Design review of the part built by this model. Coordinates are the model's own, in mm. Face numbers are marked on the shaded views. A direction names the side the tool comes from. Coordinates: 2 decimals unless noted, no trailing zeros. Loops run counter-clockwise (first coordinate to the right, second up) from the corner with the lowest first, then second, coordinate; pieces in that order, holes last. Notation, with made-up numbers: M 89.25,25 L 135.25,25 A21 ccw 135.25,30 Z; hole C 53.5,52.25 d6. An arc over 180 degrees is marked long. Put each result on its own line as item: value. Start each with the question number.
(1) Take a section at A-A, the plane x = 34.1. Give the boundary of the cut face in (y, z).
(2) Take a section at B-B, the plane y = 24.1. Give the boundary of the cut face in (x, z).
(3) Take a section at C-C, the plane x = 40.25. Give the boundary of the cut face in (y, z), then the cut area to 3 significant figures.
(4) For probe 1 along X at (y, z) = (24.1, 1); probe 2 along Y at (x, z) = (38.25, 19); probe 3 along X at (y, z) = (17, 4.25), list the stretches that pass through material, from the lowest coordinate up. Write a range as [from, to].
(5) The part is to be moulded in two halves that separate along X. For the marked faces 1, 2 and 3, say which applies: +X half, -X half, draft (parallel to the pull), parting line (faces both ways), or undercut.
(6) Take a section at D-D, the plane z = 12.5. Give the boundary of the cut face in (x, y), then the cut area to 3 significant figures.
(7) Clearance check with flat-ended pins moving along their axes: pin 1 (1.5 mm diameter, centred on x = 26.5, y = 29.5, fed in from +Z); pin 2 (3 mm diameter, centred on x = 34.1, y = 24.1, fed in from +Z); pin 3 (6 mm diameter, centred on x = 26, y = 26, fed in from +Z); pin 4 (12 mm diameter, centred on x = 26.5, z = 12, fed in from +Y). State where each tip first meets the part, or that it passes through.
(8) For the marked faces 4 and 5, list the 3-axis set-ups (+Z, -Z, +X, -X, +Y, -Y) from which the entire face can be reached by the end or side of a thin tool; tool diameter is ignored.
```python
from build123d import *

# Parameters (mm, degrees)
PAD001_DEPTH            = 20
POCKET001_DEPTH         = 16
HOLE002_D               = 4
HOLE002_CSINK_D         = 7
HOLE002_CSINK_ANGLE     = 90
HOLE003_D               = 4.2
HOLE003_DEPTH           = 25
HOLE003_CSINK_D         = 8.1
HOLE003_CSINK_ANGLE     = 90
BODY001_PLACEMENT_ANGLE = 90


with BuildPart() as part:
    # Sketch004 → Pad001 (new body)
    with BuildSketch(Plane.XZ):
        with BuildLine():
            Line((1, 0), (19, 0))
            ThreePointArc((19, 0), (19.707107, 0.292893), (20, 1))
            Line((20, 1), (20, 2))
            ThreePointArc((20, 2), (19.92388, 2.382683), (19.707107, 2.707107))
            Line((19.707107, 2.707107), (2.707107, 19.707107))
            ThreePointArc((2.707107, 19.707107), (2.382683, 19.92388), (2, 20))
            Line((2, 20), (1, 20))
            Line((1, 20), (1, 0))
        make_face()
    extrude(amount=PAD001_DEPTH)

    # Sketch005 (on Face10 of Pad001) → Pocket001 (cut)
    with BuildSketch(Plane.XZ.offset(18)):
        with BuildLine():
            Line((3, 19), (3, 4))
            ThreePointArc((3, 4), (3.292893, 3.292893), (4, 3))
            Line((4, 3), (19, 3))
            ThreePointArc((20, 2), (19.707107, 2.707107), (19, 3))
            Line((20, 20), (20, 2))
            Line((2, 20), (20, 20))
            ThreePointArc((3, 19), (2.707107, 19.707107), (2, 20))
        make_face()
    extrude(amount=-POCKET001_DEPTH, mode=Mode.SUBTRACT)

    # Hole002 (through all)
    with Locations(Plane(origin=(0, 0, 3), x_dir=(-1, 0, 0), z_dir=(0, 0, 1))):
        with Locations((-11.5, 10)):
            CounterSinkHole(HOLE002_D / 2, HOLE002_CSINK_D / 2, counter_sink_angle=HOLE002_CSINK_ANGLE)

    # Hole003
    with Locations(Plane(origin=(3, 0, 0), x_dir=(0, 0, 1), z_dir=(1, 0, 0))):
        with Locations((12.5, 10)):
            CounterSinkHole(HOLE003_D / 2, HOLE003_CSINK_D / 2, depth=HOLE003_DEPTH, counter_sink_angle=HOLE003_CSINK_ANGLE)


with BuildPart() as part_1:
    # Body001 placement: moved
    add(part.part.moved(Location((24.1, 12.6, 0))).rotate(Axis((24.1, 12.6, 0), (0, 0, 1)), BODY001_PLACEMENT_ANGLE))


solid = part_1.part
```
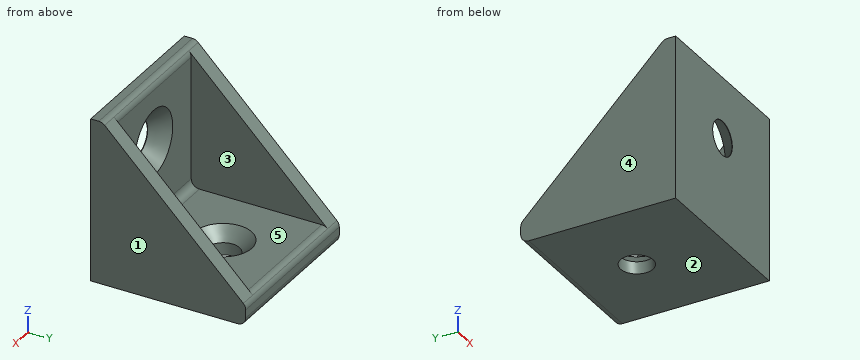
Computed values:
1. outline: M 13.6,0 L 22.1,0 L 22.1,1.5 L 20.6,3 L 16.6,3 A1 cw 15.6,4 L 15.6,8.45 L 13.65,10.4 L 13.6,10.4 Z; M 13.6,14.6 L 13.65,14.6 L 15.6,16.55 L 15.6,19 A1 ccw 14.6,20 L 13.6,20 Z; M 26.1,0 L 31.6,0 A1 ccw 32.6,1 L 32.6,2 A1 ccw 31.6,3 L 27.6,3 L 26.1,1.5 Z
2. outline: M 24.1,0 L 32.1,0 L 32.1,1.5 L 30.6,3 L 26.1,3 L 26.1,10.91 L 24.1,10.91 Z; M 36.1,0 L 44.1,0 L 44.1,10.91 L 42.1,10.91 L 42.1,3 L 37.6,3 L 36.1,1.5 Z
3. outline: M 13.6,0 L 31.6,0 A1 ccw 32.6,1 L 32.6,2 A1 ccw 31.6,3 L 16.6,3 A1 cw 15.6,4 L 15.6,19 A1 ccw 14.6,20 L 13.6,20 Z
3. area: 90.6 mm^2
4. probe 1: x = [24.1, 32.1], [36.1, 44.1]
4. probe 2: y = [13.6, 15.6]
4. probe 3: x = [24.1, 26.1], [42.1, 44.1]
5. face 1: +X half
5. face 2: draft
5. face 3: undercut
6. outline: M 24.1,13.6 L 32,13.6 L 32,13.65 L 30.05,15.6 L 26.1,15.6 L 26.1,22.51 L 24.1,22.51 Z; M 36.2,13.6 L 44.1,13.6 L 44.1,22.51 L 42.1,22.51 L 42.1,15.6 L 38.15,15.6 L 36.2,13.65 Z
6. area: 55.5 mm^2
7. pin 1: stops at z = 6.15
7. pin 2: passes through
7. pin 3: stops at z = 12.01
7. pin 4: stops at y = 29
8. face 4: +Z, -Z, -X, +Y, -Y
8. face 5: +Z, +Y
